from build123d import *

# Parameters (mm, degrees)
SKETCH2_W   = 4.1529
SKETCH2_H   = 7.1374
SKETCH2_W_2 = 5.941173797
SKETCH2_H_2 = 5.941173796
SKETCH2_H_3 = 5.941173797


with BuildPart() as part:
    # Sketch1 → Revolve1 (revolve)
    with BuildSketch(Plane.XY, mode=Mode.PRIVATE) as revolve1_sk:
        Polygon((41.1353, 50.322953291), (38.5953, 50.322953291), (14.1732, 36.222847282), (14.1732, 29.872847282), (35.6616, -50.322953291), (57.7596, -50.322953291), (41.067887421, 11.97136612), (41.1353, 12.222953291), (45.7327, 12.222953291), (45.7327, 37.622953291), (41.1353, 37.622953291), align=None)
    revolve(revolve1_sk.sketch.rotate(Axis((0, 50.322953291, 0), (0, -1, 0)), 180), axis=Axis((0, 50.322953291, 0), (0, -1, 0)))

    # Sketch2 → Cut-Revolve1 (revolve, cut)
    with BuildSketch(Plane.XY, mode=Mode.PRIVATE) as cut_revolve1_sk:
        with Locations((39.05885, 43.972953291)):
            Rectangle(SKETCH2_W, SKETCH2_H)
        with Locations((42.762113102, 29.572366393)):
            Rectangle(SKETCH2_W_2, SKETCH2_H_2)
        with Locations((42.762113102, 20.27354019)):
            Rectangle(SKETCH2_W_2, SKETCH2_H_3)
    revolve(cut_revolve1_sk.sketch.rotate(Axis((0, 50.322953291, 0), (0, 1, 0)), 180), axis=Axis((0, 50.322953291, 0), (0, 1, 0)), mode=Mode.SUBTRACT)


solid = part.part
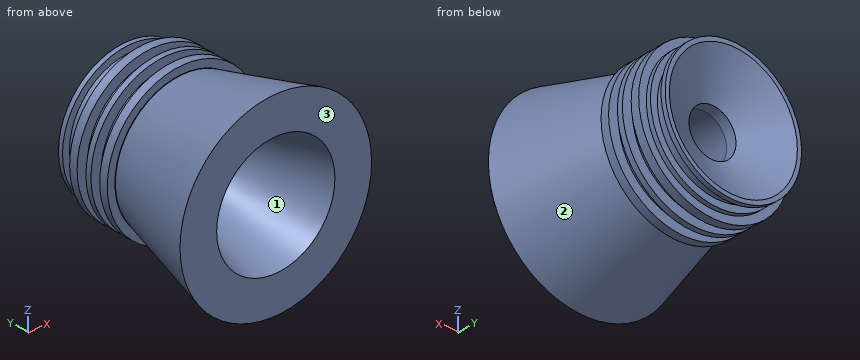
Design review of the part built by this model. Coordinates are the model's own, in mm. Face numbers are marked on the shaded views. Round coordinates to 2 decimals unless told otherwise and drop trailing zeros. Write each loop counter-clockwise with the first axis right and the second up, starting at its lowest first coordinate (ties: lowest second). Pieces come first, ordered by that corner, then holes.
Item 1: For pin 1 Ø1.5 at (x, y) = (6, -35.5) entering from -Z; pin 2 Ø24.5 at (x, z) = (5.5, 15) entering from +Y; pin 3 Ø6 at (x, y) = (6.5, 16.5) entering from -Z, all flat-tipped, find the tip position at first contact; note any pin that passes through.
Item 2: Wall thickness on L1, parallel to Y at x = -33.5, z = 23; L2, parallel to Z at x = 0, y = 32; L3, parallel to Z at x = 0, y = 32.75: over which ranges is each line inside the solid? List them lowest first.
Item 3: Consider section B-B on y = -44. Give the boundary of the cut face in (x, z).
Item 4: Consider section A-A on y = -14. Give the boundary of the cut face in (x, z), and give its area (3 significant figures).
Item 5: Draft analysis for pull direction Z (two halves, no side actions). For the marked faces 1, 2 and 3, state which applies: released by +Z, released by -Z, zero draft, split by the parting line, or undercut.
Check values:
1. pin 1: stops at z = -53.67
1. pin 2: stops at y = 44.34
1. pin 3: stops at z = -45.6
2. L1: y = -50.32 to 17.3, 23.24 to 26.6, 32.54 to 40.4, 47.54 to 50.32
2. L2: z = -39.79 to -14.17, 14.17 to 39.79
2. L3: z = -45.73 to -14.17, 14.17 to 45.73
3. outline: circle Ø112.13 at (0, 0); hole circle Ø67.93 at (0, 0)
4. outline: circle Ø96.05 at (0, 0); hole circle Ø51.86 at (0, 0)
4. area: 5,130 mm2
5. face 1: undercut
5. face 2: split by the parting line
5. face 3: zero draft
